from build123d import *

# Parameters (mm, degrees)
F0_W     = 25.4
F0_H     = 3.358979
F1_DEPTH = 25.4
F3_DEPTH = 4.445
F4_W     = 1.742139
F4_H     = 18.292457
F5_DEPTH = 4.445


with BuildPart() as f1:
    # F0 (on Front) → F1 (new body)
    with BuildSketch(Plane.XZ):
        with Locations((1.297712, -1.679489)):
            Rectangle(F0_W, F0_H)
    extrude(amount=F1_DEPTH)

    # F2 (on Top) → F3 (join)
    with BuildSketch(Plane.XY):
        Polygon((-10.09671, -1.113531), (-11.425932, 0), (-11.425932, -25.514245), (-10.09671, -24.279967), align=None)
        Polygon((14.01917, 0), (-11.425932, 0), (-10.09671, -1.113531), (12.689948, -1.113531), align=None)
        Polygon((14.01917, -25.514245), (14.01917, 0), (12.689948, -1.113531), (12.689948, -24.279967), align=None)
        Polygon((-10.09671, -24.279967), (-11.425932, -25.514245), (14.01917, -25.514245), (12.689948, -24.279967), align=None)
    extrude(amount=F3_DEPTH)

    # F4 (on Top) → F5 (join)
    with BuildSketch(Plane.XY):
        with Locations((-7.166284, -13.211324)):
            Rectangle(F4_W, F4_H)
        Polygon((7.766334, -4.065096), (0, -4.065096), (-4.801954, -4.065096), (-4.801954, -22.357553), (-3.433129, -22.357553), (-3.433129, -6.802742), (7.766334, -6.802742), align=None)
        Polygon((1.41997, -9.664828), (0, -9.664828), (0, -22.357553), (9.757349, -22.357553), (9.757349, -20.615416), (1.41997, -20.615416), align=None)
        Polygon((8.512964, -11.15809), (8.512964, -8.296004), (2.788794, -8.296004), (2.788794, -18.997714), (8.139649, -18.997714), (8.139649, -17.628891), (4.157616, -17.628891), (4.157616, -11.15809), align=None)
    extrude(amount=F5_DEPTH)


solid = f1.part
Design review of the part built by this model. Coordinates are the model's own, in mm. A direction names the side the tool comes from. Round coordinates to 2 decimals unless told otherwise and drop trailing zeros. Order: outer loops, then holes, each group sorted by start corner. A loop starts at its lowest first (then second) coordinate and runs counter-clockwise, first axis right, second up. Notation, with made-up numbers: M 32.25,42 L 65.25,42 A7 cw 65.25,46 Z; hole C 49.5,30.5 d3. An arc over 180 degrees is marked long. Answer as CSV lines item,"result". Start each with the question number.
1) Add section A-A (z = 2.25). Give the number of separate pieces and of enclosed holes in the cut face, then the cut area to 3 significant figures.
2) Add section D-D (x = -5.25). Give the boundary of the cut face in (y, z) (3 decimals).
3) Wall thickness on line 1 along X through (y, z) = (-20, 3.75); line 2 along Y through (x, z) = (3.25, 0.75); line 3 along Y through (x, z) = (9, 3): over which ranges is each line inside the solid? List them lowest first. Write a range as [from, to].
4) The part is to be moulded in two halves that separate along X. For faces 3 (the face through (1, 0, 0)), 4 (the face through (5, -22.358, 2)), 5 (the face through (-4, -22.358, 2)), 6 (the face through (-11.402, -13, -2)), say which applies: +X half, -X half, draft (parallel to the pull), parting line (faces both ways), or undercut.
5) Add section B-B (x = 2). Give the boundary of the cut face in (y, z) (3 decimals), then the cut area to 3 significant figures.
6) Tool access review of faces 1 (the face through (1, -25.514, 2)), 2 (the face through (9.757, -21, 2)): name each direction out of +Z, -Z, +X, -X, +Y, -Y from which nothing blocks a thin tool from reaching the whole face with its end or side.
7) For pin 1 Ø1.7 at (y, z) = (-7, -2) entering from -X; pin 2 Ø2 at (x, z) = (4, 2.5) entering from +Y, all flat-tipped, find the tip position at first contact; note any pin that passes through.
8) Add section C-C (y = -21.5). Give the boundary of the cut face in (x, z) (3 decimals), then the cut area to 3 significant figures.
Resolved:
1,separate pieces,"5"
1,enclosed holes,"1"
1,area,"274 mm^2"
2,outline,"M -25.514,0 L -25.4,0 L -25.4,-3.359 L 0,-3.359 L 0,4.445 L -1.114,4.445 L -1.114,0 L -24.28,0 L -24.28,4.445 L -25.514,4.445 Z"
3,line 1,"[-11.43, -10.1], [-8.04, -6.3], [-4.8, -3.43], [0, 1.42], [12.69, 14.02]"
3,line 2,"[-25.51, -24.28], [-22.36, -20.62], [-19, -8.3], [-6.8, -4.07], [-1.11, 0]"
3,line 3,"[-25.51, -24.28], [-22.36, -20.62], [-1.11, 0]"
4,face 3,"draft"
4,face 4,"undercut"
4,face 5,"undercut"
4,face 6,"-X half"
5,outline,"M -25.514,0 L -25.4,0 L -25.4,-3.359 L 0,-3.359 L 0,4.445 L -1.114,4.445 L -1.114,0 L -4.065,0 L -4.065,4.445 L -6.803,4.445 L -6.803,0 L -20.615,0 L -20.615,4.445 L -22.358,4.445 L -22.358,0 L -24.28,0 L -24.28,4.445 L -25.514,4.445 Z"
5,area,"116 mm^2"
6,face 1,"+Z, -Z, +X, -X, -Y"
6,face 2,"+Z"
7,pin 1,"x = -11.4"
7,pin 2,"y = 0"
8,outline,"M -11.426,0 L -11.402,0 L -11.402,-3.359 L 13.998,-3.359 L 13.998,0 L 14.019,0 L 14.019,4.445 L 12.69,4.445 L 12.69,0 L 9.757,0 L 9.757,4.445 L 0,4.445 L 0,0 L -3.433,0 L -3.433,4.445 L -4.802,4.445 L -4.802,0 L -6.295,0 L -6.295,4.445 L -8.037,4.445 L -8.037,0 L -10.097,0 L -10.097,4.445 L -11.426,4.445 Z"
8,area,"154 mm^2"
